Here's how the part is built. I have some questions about the finished solid (model axes, mm). Coordinates: 2 decimals unless noted, no trailing zeros. Order: outer loops, then holes, each group sorted by start corner. A loop starts at its lowest first (then second) coordinate and runs counter-clockwise, first axis right, second up. Notation, with made-up numbers: (21, 39.25) - (27, 39.25) arc R17 cw to (27, 72.25) - close; hole circle Ø11 at (55.5, 88.25). An arc over 180 degrees is marked (long way). Answer as CSV lines item,"result". Start each with the question number.
Item 1: Imagine slicing it at D-D on y = 19.5. List the corners of the cut face in (x, z) for me, and give its area (3 significant figures).
Item 2: Imagine slicing it at B-B on x = 33. List the corners of the cut face in (y, z) for me, and give its area (3 significant figures).
Item 3: Imagine slicing it at C-C on z = 16.5. List the corners of the cut face in (x, y) for me, and give its area (3 significant figures).
Item 4: I need wall thicknesses on line 1 (Y direction, x = 53, z = 32); line 2 (X direction, y = 13.25, z = 6); line 3 (Z direction, x = 53.1, y = 12.5). Which ranges of each line are inside material? Lowest first, please.
Item 5: We'd pull the mould along Y, two halves only. Please class faces 1 (the face through (54, 13, 19)), 2 (the face through (31.5, 12.43, 0.99)), 3 (the face through (23.8, 0, 1.7)), 4 (the face through (53.014, 12.775, 44.497)): pulls with the +Y half, pulls with the -Y half, needs draft (parallel to the pull), parting line crosses it, or undercut.
Item 6: Imagine slicing it at A-A on z = 25. List the corners of the cut face in (x, y) for me.
Item 7: I'm going to push a flat-ended pin straight in: pin 1 (5 mm diameter, centred on x = 17.5, y = 16, fed in from +Z). Where does the tip first touch, or does it pass through?
Autodesk Inventor part; units mm, degrees
ref_plane "YZ Plane" through (0, 0, 0) normal (1, 0, 0) x (0, 1, 0)
ref_plane "XZ Plane" through (0, 0, 0) normal (0, 1, 0) x (-1, 0, 0)
ref_plane "XY Plane" through (0, 0, 0) normal (0, 0, 1) x (1, 0, 0)
sketch "Sketch1" plane through (0, 0, 0) normal (0, 0, 1) x (1, 0, 0)
  line L0 (0, 0) -> (52, 0)
  line L1 (52, 0) -> (52, 25)
  line L2 (52, 25) -> (0, 25)
  line L3 (0, 25) -> (0, 0)
  circle A0 centre (26, 19.5) radius 1.5
  circle A1 centre (19, 12.5) radius 1.5
  circle A2 centre (33, 12.5) radius 1.5
  circle A3 centre (26, 5.5) radius 1.5
  circle A4 centre (7.4, 12.5) radius 1.5
  circle A5 centre (44.6, 12.5) radius 1.5
  circle A6 centre (26, 12.5) radius 4.0289
  line L4 (52, 25) -> (54, 25)
  line L5 (54, 25) -> (54, 0)
  line L6 (54, 0) -> (52, 0)
  line L7 (52, 0) -> (52, 25)
  line L8 (0, 25) -> (-2, 25)
  line L9 (-2, 25) -> (-2, 0)
  line L10 (-2, 0) -> (0, 0)
  line L11 (0, 0) -> (0, 25)
  dimension "d0" = 52
  dimension "d1" = 25
  dimension "d2" = 3
  dimension "d3" = 3
  dimension "d4" = 3
  dimension "d5" = 3
  dimension "d6" = 3
  dimension "d7" = 3
  dimension "d9" = 7.4
  dimension "d10" = 7.4
  dimension "d11" = 26
  dimension "d13" = 2
  dimension "d14" = 2
extrude "Extrusion1" add sketch "Sketch1" along normal blind 2 contours L3 L2 L1 L0
extrude "Extrusion2" add sketch "Sketch1" along normal blind 3 contours L10 L9 L8 L3 | L1 L4 L5 L6
sketch "Sketch2" plane through (0, 0, 3) normal (0, 0, 1) x (1, 0, 0)
  line L0 (54, 25) -> (-2, 25)
  line L1 (0, 0) -> (0, 25)
  line L2 (-2, 25) -> (0, 25)
  line L3 (0, 25) -> (0, 0)
  line L4 (0, 0) -> (-2, 0)
  line L5 (-2, 0) -> (-2, 25)
  line L6 (52, 25) -> (52, 0)
  line L7 (54, 0) -> (54, 25)
  line L8 (52, 25) -> (54, 25)
  line L9 (54, 25) -> (54, 0)
  line L10 (54, 0) -> (52, 0)
  line L11 (52, 0) -> (52, 25)
extrude "Extrusion3" add sketch "Sketch2" along normal blind 29
sketch "Sketch3" plane through (54, 0, 0) normal (1, 0, 0) x (0, 0, -1)
  line L0 (-32, 0) -> (-32, 25)
  line L1 (-2, 25) -> (-32, 25)
  line L2 (-2, 0) -> (-32, 0)
  arc A0 (-32, 25) -> (-32, 0) centre (-32, 12.5) ccw
  line L3 (-32, 0) -> (-32, 25)
  point P0 (0, 0)
  dimension "d22" = 12.5
extrude "Extrusion4" add sketch "Sketch3" against normal blind 2
sketch "Sketch4" plane through (-2, 0, 0) normal (-1, 0, 0) x (0, 0, 1)
  arc A0 (32, 0) -> (32, 25) centre (32, 12.5) ccw
  line L0 (2, 25) -> (32, 25)
  arc A1 (32, 0) -> (32, 25) centre (32, 12.5) ccw
  line L1 (32, 25) -> (32, 0)
  point P0 (0, 0)
extrude "Extrusion5" add sketch "Sketch4" against normal blind 2
fillet "Fillet1" radius 2 2 edges at (54, 12.5, 0) (-2, 12.5, 0)
sketch "Sketch5" plane through (-2, 12.5, 32) normal (-1, 0, 0) x (0, 0, 1)
  circle A0 centre (0, 0) radius 4
  circle A1 centre (0, 0) radius 7
  circle A2 centre (0, 7) radius 1.5
  circle A3 centre (-7, 0) radius 1.5
  circle A4 centre (0, -7) radius 1.5
  circle A5 centre (7, 0) radius 1.5
  circle A6 centre (-18.6, 0) radius 1.3978
  point P0 (-32, -12.5)
  dimension "d29" = 14
  dimension "d28" = 8
  dimension "d32" = 360
  dimension "d34" = 3
  dimension "d35" = 18.6
hole "Hole1" at (-2, 12.5, 32) at (-2, 12.5, 25) at (-2, 19.5, 32) at (-2, 12.5, 39) at (-2, 5.5, 32) at (-2, 12.5, 13.4) direction (1, 0, 0) diameter 3 end through all
hole "Hole2" at (-2, 12.5, 32) direction (1, 0, 0) diameter 8 end through all
properties part number "Bracket U CORTO"
Responses:
1,outline,"(-2, 2) arc R2 ccw to (0, 0) - (24.5, 0) - (24.5, 2) - (0, 2) - (0, 30.5) - (-2, 30.5) - close; (-2, 33.5) - (0, 33.5) - (0, 42.36) - (-2, 42.36) - close; (27.5, 0) - (52, 0) arc R2 ccw to (54, 2) - (54, 30.5) - (52, 30.5) - (52, 2) - (27.5, 2) - close; (52, 33.5) - (54, 33.5) - (54, 42.36) - (52, 42.36) - close"
1,area,"254 mm^2"
2,outline,"(0, 0) - (11, 0) - (11, 2) - (0, 2) - close; (14, 0) - (25, 0) - (25, 2) - (14, 2) - close"
2,area,"44.0 mm^2"
3,outline,"(-2, 0) - (0, 0) - (0, 25) - (-2, 25) - close; (52, 0) - (54, 0) - (54, 25) - (52, 25) - close"
3,area,"100 mm^2"
4,line 1,"y = 0 to 4, 7 to 8.5, 16.5 to 18, 21 to 25"
4,line 2,"x = -2 to 0, 52 to 54"
4,line 3,"z = 0.33 to 11.9, 14.9 to 23.5, 26.5 to 28, 36 to 37.5, 40.5 to 44.5"
5,face 1,"needs draft"
5,face 2,"undercut"
5,face 3,"pulls with the -Y half"
5,face 4,"parting line crosses it"
6,outline,"(-2, 0) - (0, 0) - (0, 11) - (-2, 11) - close; (-2, 14) - (0, 14) - (0, 25) - (-2, 25) - close; (52, 0) - (54, 0) - (54, 11) - (52, 11) - close; (52, 14) - (54, 14) - (54, 25) - (52, 25) - close"
7,pin 1,"stops at z = 2"
